Could you check a few things on this model? Use its own coordinates, in mm. Face numbers are marked on the shaded views. A direction names the side the tool comes from. Coordinates: 2 decimals unless noted, no trailing zeros. Write each loop counter-clockwise with the first axis right and the second up, starting at its lowest first coordinate (ties: lowest second). Pieces come first, ordered by that corner, then holes.
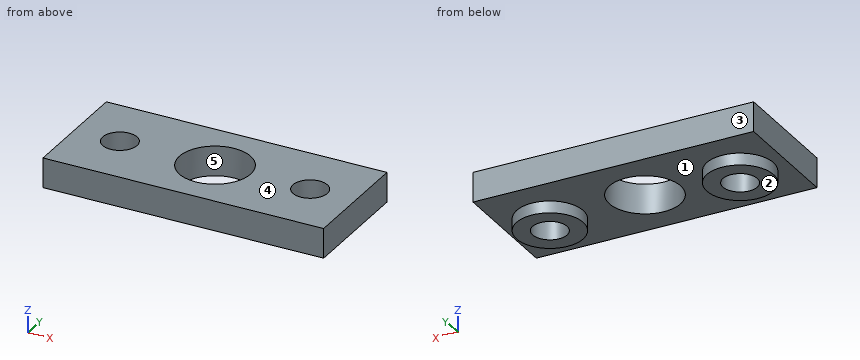
```python
from build123d import *

# Parameters (mm, degrees)
SKETCH_1_W                             = 23.6
SKETCH_1_H                             = 10
SKETCH_1_R                             = 1.45
SKETCH_1_R_2                           = 3
PLATE_23_6X10_T2_5_M2_5_D2_9_P16_DEPTH = 2.5
UNIT_RECESS_RINGS_OD5_6_ID2_9_H1_START = -1
SKETCH_2_R                             = 2.8
SKETCH_2_R_2                           = 1.45
UNIT_RECESS_RINGS_OD5_6_ID2_9_H1_DEPTH = 1


with BuildPart() as part:
    # 草图1 → Plate_23.6x10_T2.5_M2.5_D2.9_P16 (new body)
    with BuildSketch(Plane.XY):
        Rectangle(SKETCH_1_W, SKETCH_1_H)
        with Locations((-8, 0)):
            Circle(SKETCH_1_R, mode=Mode.SUBTRACT)
        with Locations((8, 0)):
            Circle(SKETCH_1_R, mode=Mode.SUBTRACT)
        Circle(SKETCH_1_R_2, mode=Mode.SUBTRACT)
    extrude(amount=PLATE_23_6X10_T2_5_M2_5_D2_9_P16_DEPTH)

    # 草图2 → Unit_recess_rings_OD5.6_ID2.9_H1 (add)
    # profile 1 of 2: a face of its own
    with BuildSketch(Plane.XY.offset(UNIT_RECESS_RINGS_OD5_6_ID2_9_H1_START)):
        with Locations((-8, 0)):
            Circle(SKETCH_2_R)
        with Locations((-8, 0)):
            Circle(SKETCH_2_R_2, mode=Mode.SUBTRACT)
    # profile 2 of 2: a face of its own
    with BuildSketch(Plane.XY.offset(UNIT_RECESS_RINGS_OD5_6_ID2_9_H1_START)):
        with Locations((8, 0)):
            Circle(SKETCH_2_R)
        with Locations((8, 0)):
            Circle(SKETCH_2_R_2, mode=Mode.SUBTRACT)
    extrude(amount=UNIT_RECESS_RINGS_OD5_6_ID2_9_H1_DEPTH)


solid = part.part
```
Item 1: I want a section at B-B, the plane x = -8. List the corners of the cut face in (y, z) for me.
Item 2: If we mould it in two halves opening along Y, with no side actions, what happens to the marked faces 3, 4 and 5? For each: released by +Y, released by -Y, zero draft, split by the parting line, or undercut.
Item 3: Which directions (+Z, -Z, +X, -X, +Y, -Y) give clear straight access to the entire face, cutting with the end or side of a thin tool? Please do the marked faces 1 and 2.
Item 4: I want a section at D-D, the plane y = -2. List the corners of the cut face in (x, z) for me.
Item 5: If I drill on line 1 along Y through (x, z) = (0, 0.8); line 2 along X through (y, z) = (-1, 2); line 3 along Z through (x, y) = (1, 4.5), over which ranges is the centre line in solid material (lowest first)?
Item 6: I want a section at C-C, the plane z = 1.2. List the corners of the cut face in (x, y) for me, then the cut area to 3 significant figures.
Item 7: I want a section at A-A, the plane y = 0. List the corners of the cut face in (x, z) for me.
Taken from the geometry:
1. outline: (-5, 0) - (-2.8, 0) - (-2.8, -1) - (-1.45, -1) - (-1.45, 2.5) - (-5, 2.5) - close; (1.45, -1) - (2.8, -1) - (2.8, 0) - (5, 0) - (5, 2.5) - (1.45, 2.5) - close
2. face 3: released by +Y
2. face 4: zero draft
2. face 5: undercut
3. face 1: -Z
3. face 2: -Z, +X, -X, +Y, -Y
4. outline: (-11.8, 0) - (-9.96, 0) - (-9.96, -1) - (-6.04, -1) - (-6.04, 0) - (-2.24, 0) - (-2.24, 2.5) - (-11.8, 2.5) - close; (2.24, 0) - (6.04, 0) - (6.04, -1) - (9.96, -1) - (9.96, 0) - (11.8, 0) - (11.8, 2.5) - (2.24, 2.5) - close
5. line 1: y = -5 to -3, 3 to 5
5. line 2: x = -11.8 to -9.05, -6.95 to -2.83, 2.83 to 6.95, 9.05 to 11.8
5. line 3: z = 0 to 2.5
6. outline: (-11.8, -5) - (11.8, -5) - (11.8, 5) - (-11.8, 5) - close; hole circle Ø2.9 at (-8, 0); hole circle Ø6 at (0, 0); hole circle Ø2.9 at (8, 0)
6. area: 195 mm2
7. outline: (-11.8, 0) - (-10.8, 0) - (-10.8, -1) - (-9.45, -1) - (-9.45, 2.5) - (-11.8, 2.5) - close; (-6.55, -1) - (-5.2, -1) - (-5.2, 0) - (-3, 0) - (-3, 2.5) - (-6.55, 2.5) - close; (3, 0) - (5.2, 0) - (5.2, -1) - (6.55, -1) - (6.55, 2.5) - (3, 2.5) - close; (9.45, -1) - (10.8, -1) - (10.8, 0) - (11.8, 0) - (11.8, 2.5) - (9.45, 2.5) - close
